```python
from build123d import *

# Parameters (mm, degrees)
F0_R     = 7.62
F0_R_2   = 1.0795
F1_DEPTH = 12.7
F2_DEPTH = 10.16
F3_R     = 1.016


with BuildPart() as f1:
    # F0 (on Right) → F1 (new body, symmetric)
    with BuildSketch(Plane.YZ):
        Circle(F0_R)
        Circle(F0_R_2, mode=Mode.SUBTRACT)
    extrude(amount=F1_DEPTH, both=True)

    # F0 (on Right) → F2 (join, symmetric)
    with BuildSketch(Plane.YZ):
        Circle(F0_R_2)
    extrude(amount=F2_DEPTH, both=True)

    # F3
    f3_edges = [f1.edges().sort_by_distance(p)[0] for p in [
        (12.7, -7.62, 0),
        (-12.7, -7.62, 0),
    ]]
    fillet(f3_edges, radius=F3_R)


solid = f1.part
```
Verification items for the finished model (mm, model axes). A direction names the side the tool comes from. Coordinates: 2 decimals unless noted, no trailing zeros. Loops run counter-clockwise (first coordinate to the right, second up) from the corner with the lowest first, then second, coordinate; pieces in that order, holes last. Notation, with made-up numbers: (34, 65) - (73, 65) arc R13 cw to (73, 77) - close; hole circle Ø8 at (34, 18). An arc over 180 degrees is marked (long way). Answer as a JSON object with one key per item and string values.
(1) Cross-section at B-B, the plane x = -2. Record the boundary of the cut face in (y, z), then the cut area to 3 significant figures.
Response:
{"outline": "circle Ø15.24 at (0, 0)", "area": "182 mm²"}
(2) Go/stop test with flat-tipped pins: pin 1 Ø3 at (x, z) = (4.5, 3) entering from -Y; pin 2 Ø1.7 at (y, z) = (0, 0) entering from -X; pin 3 Ø3 at (x, z) = (4, 3) entering from +Y. Record where each tip stops, or that it passes through.
Response:
{"pin 1": "stops at y = -7.47", "pin 2": "stops at x = -10.16", "pin 3": "stops at y = 7.47"}
(3) Mould release check, pull along Z, two halves, no side actions. Record for faces 4 (the cylindrical face through (0.16, -1.65, -7.44)), 5 (the flat face through (12.7, -0.1, -1.4)), 6 (the flat face through (-10.16, 0, 0)): pulls with the +Z half, pulls with the -Z half, needs draft (parallel to the pull), parting line crosses it, or undercut.
Response:
{"face 4": "parting line crosses it", "face 5": "needs draft", "face 6": "undercut"}
(4) Scan lines: line 1 along Z through (x, y) = (11.55, 0); line 2 along Y through (x, z) = (0, -4.5); line 3 along X through (y, z) = (-4.75, -5.25). Record each from-to range of solid material in increasing order.
Response:
{"line 1": "z = -7.62 to -1.08, 1.08 to 7.62", "line 2": "y = -6.15 to 6.15", "line 3": "x = -12.58 to 12.58"}
(5) Access from +Z, -Z, +X, -X, +Y, -Y to the whole of each face (thin tool, end or side, straight path). Record for faces 1 (the flat face through (10.16, 0, 0)), 2 (the cylindrical face through (-11.45, -0.14, 1.07)), 3 (the flat face through (-12.7, -0.1, -1.4)).
Response:
{"face 1": "+X", "face 2": "-X", "face 3": "+Z, -Z, -X, +Y, -Y"}
(6) Cross-section at A-A, the plane y = 0. Record the boundary of the cut face in (x, z), then the cut area to 3 significant figures.
Response:
{"outline": "(-12.7, -6.6) arc R1.02 ccw to (-11.68, -7.62) - (11.68, -7.62) arc R1.02 ccw to (12.7, -6.6) - (12.7, -1.08) - (10.16, -1.08) - (10.16, 1.08) - (12.7, 1.08) - (12.7, 6.6) arc R1.02 ccw to (11.68, 7.62) - (-11.68, 7.62) arc R1.02 ccw to (-12.7, 6.6) - (-12.7, 1.08) - (-10.16, 1.08) - (-10.16, -1.08) - (-12.7, -1.08) - close", "area": "375 mm²"}
